The figure shows three views and two pictorial views of one solid part (mm, origin at its lowest corner). Answer the questions. Coordinates: 2 decimals unless noted, no trailing zeros. Loops run counter-clockwise (first coordinate to the right, second up) from the corner with the lowest first, then second, coordinate; pieces in that order, holes last. Notation, with made-up numbers: M 29.25,-29.5 L 44.25,-29.5 A18 ccw 44.25,-0.5 Z; hole C -8.75,33.5 d3. An arc over 180 degrees is marked long. Answer in a Markdown table with one row per item. Add a question column.
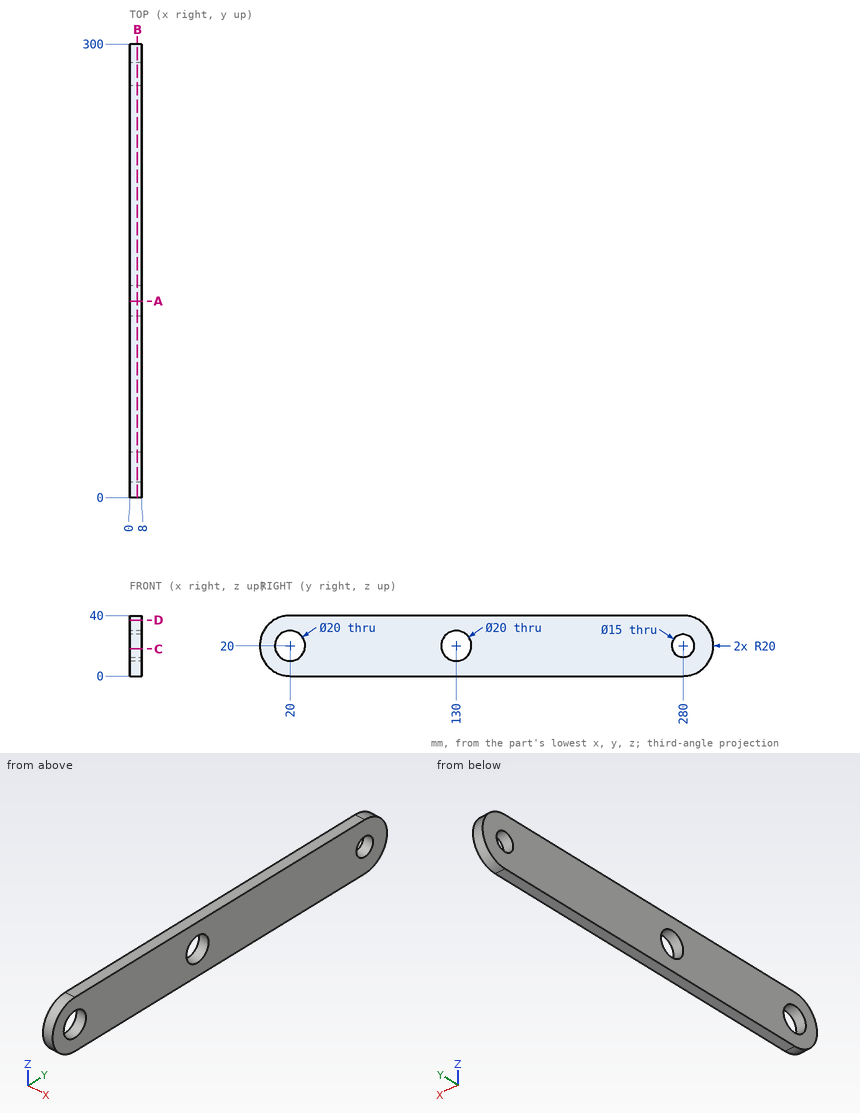
(1) Straight lines are drawn through the part: line 1 (Y direction, x = 4, z = 20); line 2 (Z direction, x = 2, y = 280); line 3 (Y direction, x = 4, z = 17.5). For each, find the intervals that lie inside material, in ascending order.
(2) A cutting plane is placed at D-D (z = 37). Give the vertices of the cut face in (x, y).
(3) A cutting plane is placed at B-B (x = 5). Give the vertices of the cut face in (y, z), plus the area to 3 significant figures.
(4) Each of these flat-tipped pins is pushed along its axis until it touches: pin 1 (3 mm diameter, centred on x = 5.5, z = 17.5, fed in from -Y) (3 decimals); pin 2 (1.5 mm diameter, centred on x = 3, z = 36, fed in from +Y). Where does it stop, or does it pass through?
(5) A cutting plane is placed at A-A (y = 130). Give the vertices of the cut face in (x, z), plus the area to 3 significant figures.
(6) A cutting plane is placed at C-C (z = 18). Give the vertices of the cut face in (x, y).
Solved:
| question | item | result |
|---|---|---|
| 1 | line 1 | y = 0 to 10, 30 to 120, 140 to 272.5, 287.5 to 300 |
| 1 | line 2 | z = 0 to 12.5, 27.5 to 40 |
| 1 | line 3 | y = 0.16 to 10.32, 29.68 to 120.32, 139.68 to 272.93, 287.07 to 299.84 |
| 2 | outline | M 0,9.46 L 8,9.46 L 8,290.54 L 0,290.54 Z |
| 3 | outline | M 20,0 L 280,0 A20 ccw 280,40 L 20,40 A20 ccw Z; hole C 20,20 d20; hole C 130,20 d20; hole C 280,20 d15 |
| 3 | area | 10,900 mm² |
| 4 | pin 1 | stops at y = 0.025 |
| 4 | pin 2 | stops at y = 292.94 |
| 5 | outline | M 0,0 L 8,0 L 8,10 L 0,10 Z; M 0,30 L 8,30 L 8,40 L 0,40 Z |
| 5 | area | 160 mm² |
| 6 | outline | M 0,0.1 L 8,0.1 L 8,10.2 L 0,10.2 Z; M 0,29.8 L 8,29.8 L 8,120.2 L 0,120.2 Z; M 0,139.8 L 8,139.8 L 8,272.77 L 0,272.77 Z; M 0,287.23 L 8,287.23 L 8,299.9 L 0,299.9 Z |
